Job drawing, mm, ordinate dimensions from the low corner. One solid piece. Give positions to 0.01 mm unless a question says otherwise; leave off trailing zeros. Loops run counter-clockwise (first coordinate to the right, second up) from the corner with the lowest first, then second, coordinate; pieces in that order, holes last. Notation, with made-up numbers: (68, -38.5) -> (95, -38.5) arc R15 ccw to (95, -14.5) -> close; hole circle Ø6 at (88, 74.25). An arc over 180 degrees is marked (long way). Answer as a JSON object with one key per item and string values. Group by question number.
Q1. Band-saw the part on D-D, the plane x = 15.5. Write the cut outline in (y, z), plus the area to 3 significant figures.
Q2. Wall check: probe 1 along X at (y, z) = (3.2, 74.5); probe 2 along Z at (x, y) = (119, 4.6); probe 3 along Z at (x, y) = (122, 3.2). Give the ranges that are in metal, low to high. Write a range as from..to.
Q3. Drop a flat-ended pin along its axis: pin 1 (3 mm diameter, centred on x = 70.5, y = 3, fed in from +Z). Give the stop position or say it passes through.
Q4. Band-saw the part on B-B, the plane z = 24. Write the cut outline in (x, y).
Q5. Band-saw the part on A-A, the plane y = 3.85. Write the cut outline in (x, z), plus the area to 3 significant figures.
Q6. Band-saw the part on C-C, the plane x = 61.5. Write the cut outline in (y, z).
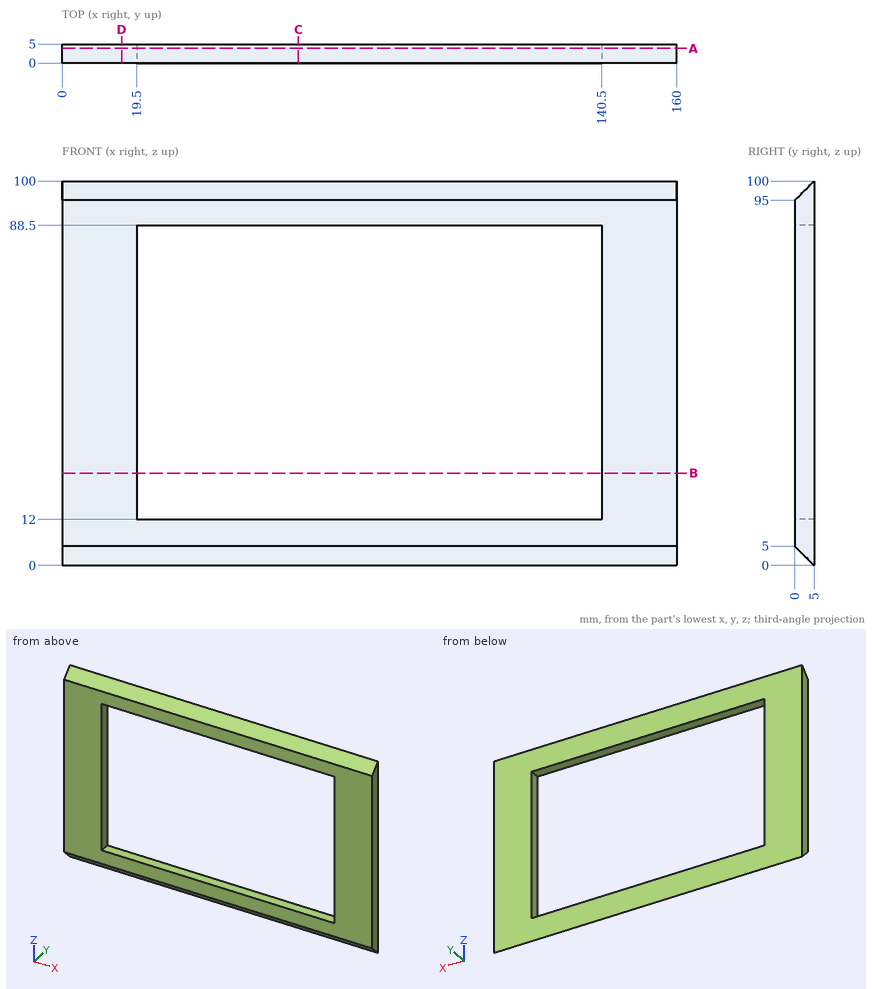
Worked answers:
{
 "1": {"outline": "(0, 5) -> (5, 0) -> (5, 100) -> (0, 95) -> close", "area": "475 mm2"},
 "2": {"probe 1": "0..19.5, 140.5..160", "probe 2": "0.4..12, 88.5..99.6", "probe 3": "1.8..12, 88.5..98.2"},
 "3": {"pin 1": "z = 99.5"},
 "4": {"outline": "(0, 0) -> (19.5, 0) -> (19.5, 5) -> (0, 5) -> close; (140.5, 0) -> (160, 0) -> (160, 5) -> (140.5, 5) -> close"},
 "5": {"outline": "(0, 1.15) -> (160, 1.15) -> (160, 98.85) -> (0, 98.85) -> close; hole (19.5, 12) -> (140.5, 12) -> (140.5, 88.5) -> (19.5, 88.5) -> close", "area": "6,380 mm2"},
 "6": {"outline": "(0, 5) -> (5, 0) -> (5, 12) -> (0, 12) -> close; (0, 88.5) -> (5, 88.5) -> (5, 100) -> (0, 95) -> close"}
}
